Could you check a few things on this model? Use its own coordinates, in mm. Round coordinates to 2 decimals unless told otherwise and drop trailing zeros. Loops run counter-clockwise (first coordinate to the right, second up) from the corner with the lowest first, then second, coordinate; pieces in that order, holes last. Notation, with made-up numbers: M 57,33.25 L 74,33.25 A23 cw 74,70.25 Z; hole C -27.75,5 d7. An arc over 180 degrees is marked long. Answer in a Markdown table with one row per item.
```python
from build123d import *

# Parameters (mm, degrees)
SKETCH_W               = 84
SKETCH_H               = 15
PAD_DEPTH              = 12
SKETCH001_R            = 8.25
POCKET_DEPTH           = 12.001
LINEARPATTERN001_COUNT = 3
LINEARPATTERN001_PITCH = 28
HOLE_D                 = 5
HOLE_CSINK_D           = 11
HOLE_CSINK_ANGLE       = 90
LINEARPATTERN_COUNT    = 2
LINEARPATTERN_PITCH    = 28


with BuildPart() as part:
    # Sketch → Pad (new body)
    with BuildSketch(Plane.XY):
        with Locations((42, 7.5)):
            Rectangle(SKETCH_W, SKETCH_H)
    extrude(amount=PAD_DEPTH)

    # Sketch001 (on DatumPlane) → Pocket (cut, through all)
    with BuildSketch(Plane.XY.offset(12)):
        with Locations((14, 15)):
            Circle(SKETCH001_R)
    pocket = extrude(amount=-POCKET_DEPTH, mode=Mode.SUBTRACT)

    # LinearPattern001: Pocket ×3
    with Locations(*[(i * LINEARPATTERN001_PITCH, 0, 0) for i in range(1, LINEARPATTERN001_COUNT)]):
        add(pocket, mode=Mode.SUBTRACT)

    # Hole (through all)
    with Locations(Plane.XZ):
        with Locations((28, 6)):
            hole = CounterSinkHole(HOLE_D / 2, HOLE_CSINK_D / 2, counter_sink_angle=HOLE_CSINK_ANGLE)

    # LinearPattern: Hole ×2
    with Locations(*[(i * LINEARPATTERN_PITCH, 0, 0) for i in range(1, LINEARPATTERN_COUNT)]):
        add(hole, mode=Mode.SUBTRACT)


solid = part.part
```
1) I need wall thicknesses on line 1 (X direction, y = 12.75, z = 6); line 2 (Z direction, x = 56, y = 10.25); line 3 (X direction, y = 9.75, z = 6). Which ranges of each line are inside material? Lowest first, please.
Computed:
| item | result |
|---|---|
| line 1 | x = 0 to 6.06, 21.94 to 25.5, 30.5 to 34.06, 49.94 to 53.5, 58.5 to 62.06, 77.94 to 84 |
| line 2 | z = 0 to 3.5, 8.5 to 12 |
| line 3 | x = 0 to 7.64, 20.36 to 25.5, 30.5 to 35.64, 48.36 to 53.5, 58.5 to 63.64, 76.36 to 84 |
2) I want a section at D-D, the plane y = 4. Please give me the cut outline in (x, z), plus the area to 3 significant figures.
Computed:
| item | result |
|---|---|
| outline | M 0,0 L 84,0 L 84,12 L 0,12 Z; hole C 28,6 d5; hole C 56,6 d5 |
| area | 969 mm² |
3) I want a section at A-A, the plane y = 11.25. Please give me the cut outline in (x, z).
Computed:
| item | result |
|---|---|
| outline | M 0,0 L 6.65,0 L 6.65,12 L 0,12 Z; M 21.35,0 L 34.65,0 L 34.65,12 L 21.35,12 Z; M 49.35,0 L 62.65,0 L 62.65,12 L 49.35,12 Z; M 77.35,0 L 84,0 L 84,12 L 77.35,12 Z; hole C 28,6 d5; hole C 56,6 d5 |
4) Will these pins go through, and if not, where does the flat tip stop? P1, Ø1.5, axis at x = 39.5, z = 4, coming from the -Y side; P2, Ø4.5, axis at x = 28, z = 6, coming from the +Y side.
Computed:
| item | result |
|---|---|
| P1 | stops at y = 0 |
| P2 | passes through |
5) I want a section at C-C, the plane x = 28. Please give me the cut outline in (y, z), plus the area to 3 significant figures.
Computed:
| item | result |
|---|---|
| outline | M 0,0 L 15,0 L 15,3.5 L 3,3.5 L 0,0.5 Z; M 0,11.5 L 3,8.5 L 15,8.5 L 15,12 L 0,12 Z |
| area | 96.0 mm² |
6) I want a section at B-B, the plane z = 6. Please give me the cut outline in (x, y).
Computed:
| item | result |
|---|---|
| outline | M 0,0 L 22.5,0 L 25.5,3 L 25.5,15 L 22.25,15 A8.25 cw 5.75,15 L 0,15 Z; M 30.5,3 L 33.5,0 L 50.5,0 L 53.5,3 L 53.5,15 L 50.25,15 A8.25 cw 33.75,15 L 30.5,15 Z; M 58.5,3 L 61.5,0 L 84,0 L 84,15 L 78.25,15 A8.25 cw 61.75,15 L 58.5,15 Z |
7) If we mould it in two halves opening along X, with no side actions, what happens to faces 1 (the face through (41, 0, 6)), 2 (the face through (84, 7, 6)), 3 (the face through (0, 7, 6)), 4 (the face through (69.82, 6.75, 6.08))? For each: released by +X, released by -X, zero draft, split by the parting line, or undercut.
Computed:
| item | result |
|---|---|
| face 1 | zero draft |
| face 2 | released by +X |
| face 3 | released by -X |
| face 4 | undercut |
